from build123d import *

# Parameters (mm, degrees)
F0_R     = 65.55
F1_DEPTH = 0.6
F2_R     = 4.25
F3_DEPTH = 2.5
F4_R     = 35
F5_DEPTH = 0.601


with BuildPart() as f1:
    # F0 (on Top) → F1 (new body)
    with BuildSketch(Plane.XY):
        Circle(F0_R)
    extrude(amount=F1_DEPTH)

    # F2 (on face) → F3 (join)
    with BuildSketch(Plane.XY.offset(0.6)):
        with Locations((-36, 36)):
            Circle(F2_R)
        with Locations((36, 36)):
            Circle(F2_R)
        with Locations((36, -36)):
            Circle(F2_R)
        with Locations((-36, -36)):
            Circle(F2_R)
    extrude(amount=F3_DEPTH)

    # F4 (on face) → F5 (cut, through all)
    with BuildSketch(Plane.XY.offset(0.6)):
        Circle(F4_R)
    extrude(amount=-F5_DEPTH, mode=Mode.SUBTRACT)


solid = f1.part
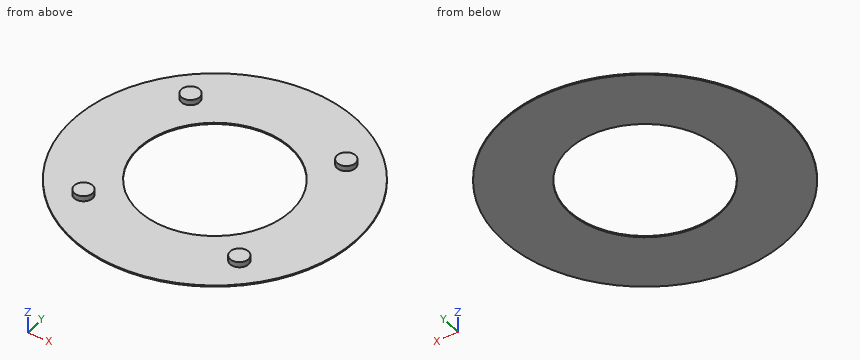
CAD build for the part. Positions are in the model's coordinates, mm. Coordinates: 2 decimals unless noted, no trailing zeros. Loops run counter-clockwise (first coordinate to the right, second up) from the corner with the lowest first, then second, coordinate; pieces in that order, holes last. Notation, with made-up numbers: (29, -39) - (34, -39) arc R8 cw to (34, -29) - close; hole circle Ø6 at (21, -17.5). An arc over 180 degrees is marked (long way). Use one line per item in the form item = value. Start each with the question number.
1) Band-saw the part on C-C (y = -25.5). Give the cut face in (x, z).
2) Band-saw the part on A-A (x = 0). Give the cut face in (y, z).
3) Drill centre lines: L1, parallel to X at y = -1, z = 0.5; L2, parallel to Y at x = 0, z = 0.3; L3, parallel to Z at x = 46, y = 29. Where is each one in solid material? Low to high. Write a range as from..to.
4) Flat gauge pin, fed straight in: pin 1 (12 mm diameter, centred on x = 1, y = 38.5, fed in from +Z). Where does the tip first touch, or does it go through?
5) Band-saw the part on D-D (x = -48). Give the cut face in (y, z), and give its area (3 significant figures).
6) Band-saw the part on B-B (z = 2.55). Give the cut face in (x, y).
Check values:
q1.outline = (-60.39, 0) - (-23.97, 0) - (-23.97, 0.6) - (-60.39, 0.6) - close; (23.97, 0) - (60.39, 0) - (60.39, 0.6) - (23.97, 0.6) - close
q2.outline = (-65.55, 0) - (-35, 0) - (-35, 0.6) - (-65.55, 0.6) - close; (35, 0) - (65.55, 0) - (65.55, 0.6) - (35, 0.6) - close
q3.L1 = -65.54..-34.99, 34.99..65.54
q3.L2 = -65.55..-35, 35..65.55
q3.L3 = 0..0.6
q4.pin_1 = 0.6
q5.outline = (-44.64, 0) - (44.64, 0) - (44.64, 0.6) - (-44.64, 0.6) - close
q5.area = 53.6 mm2
q6.outline = circle Ø8.5 at (-36, -36); circle Ø8.5 at (-36, 36); circle Ø8.5 at (36, -36); circle Ø8.5 at (36, 36)
